Model file for the job. Use its own axes, mm. A direction names the side the tool comes from. Coordinates: 2 decimals unless noted, no trailing zeros. Order: outer loops, then holes, each group sorted by start corner. A loop starts at its lowest first (then second) coordinate and runs counter-clockwise, first axis right, second up.
from build123d import *

# Parameters (mm, degrees)
SKETCH_1_R              = 3
EXTRUDE_1_DEPTH         = 1.5
SHEET_START             = -1.5
SHEET_METAL_1_OUTLINE_R = 3
SHEET_METAL_1_DEPTH     = 1.5


# Read off the part's stored shape, not the designer's step: Преобразовать-Твердое тело1
with BuildPart() as part:
    # Sketch 1 → Бобышка-Вытянуть1 (new body)
    with BuildSketch(Plane.XY):
        with BuildLine():
            Line((-75, -160), (-75, 187.455080757))
            Line((-75, 187.455080757), (-302.165063509, 187.455080757))
            Line((-302.165063509, 187.455080757), (-346.732050808, 110.262794416))
            Line((-346.732050808, 110.262794416), (-364.052558883, 120.262794416))
            Line((-364.052558883, 120.262794416), (-374.052558883, 102.942286341))
            Line((-374.052558883, 102.942286341), (-356.732050808, 92.942286341))
            Line((-356.732050808, 92.942286341), (-401.299038106, 15.75))
            ThreePointArc((-401.299038106, 15.75), (-401.700961894, 14.25), (-401.299038106, 12.75))
            Line((-401.299038106, 12.75), (-376.299038106, -30.551270189))
            Line((-376.299038106, -30.551270189), (-392.320508076, -39.801270189))
            Line((-392.320508076, -39.801270189), (-382.320508076, -57.121778265))
            Line((-382.320508076, -57.121778265), (-366.299038106, -47.871778265))
            Line((-366.299038106, -47.871778265), (-241.299038106, -264.378129211))
            Line((-241.299038106, -264.378129211), (-257.320508076, -273.628129211))
            Line((-257.320508076, -273.628129211), (-247.320508076, -290.948637287))
            Line((-247.320508076, -290.948637287), (-231.299038106, -281.698637287))
            Line((-231.299038106, -281.698637287), (-203.75277675, -329.410161514))
            ThreePointArc((-203.75277675, -329.410161514), (-200.092522712, -333.070415552), (-195.092522712, -334.410161514))
            Line((-195.092522712, -334.410161514), (-149.133974596, -334.410161514))
            Line((-149.133974596, -334.410161514), (-149.133974596, -352.910161514))
            Line((-149.133974596, -352.910161514), (-129.133974596, -352.910161514))
            Line((-129.133974596, -352.910161514), (-129.133974596, -334.410161514))
            Line((-129.133974596, -334.410161514), (129.133974596, -334.410161514))
            Line((129.133974596, -334.410161514), (129.133974596, -352.910161514))
            Line((129.133974596, -352.910161514), (149.133974596, -352.910161514))
            Line((149.133974596, -352.910161514), (149.133974596, -334.410161514))
            Line((149.133974596, -334.410161514), (195.092522712, -334.410161514))
            ThreePointArc((195.092522712, -334.410161514), (200.092522712, -333.070415552), (203.75277675, -329.410161514))
            Line((203.75277675, -329.410161514), (231.299038106, -281.698637287))
            Line((231.299038106, -281.698637287), (247.320508076, -290.948637287))
            Line((247.320508076, -290.948637287), (257.320508076, -273.628129211))
            Line((257.320508076, -273.628129211), (241.299038106, -264.378129211))
            Line((241.299038106, -264.378129211), (366.299038106, -47.871778265))
            Line((366.299038106, -47.871778265), (382.320508076, -57.121778265))
            Line((382.320508076, -57.121778265), (392.320508076, -39.801270189))
            Line((392.320508076, -39.801270189), (376.299038106, -30.551270189))
            Line((376.299038106, -30.551270189), (401.299038106, 12.75))
            ThreePointArc((401.299038106, 12.75), (401.700961894, 14.25), (401.299038106, 15.75))
            Line((401.299038106, 15.75), (302.165063509, 187.455080757))
            Line((302.165063509, 187.455080757), (75, 187.455080757))
            Line((75, 187.455080757), (75, -160))
            ThreePointArc((75, -160), (0, -235), (-75, -160))
        make_face()
        with Locations((244.309773091, -277.663383249)):
            Circle(SKETCH_1_R, mode=Mode.SUBTRACT)
        with Locations((139.133974596, -343.660161514)):
            Circle(SKETCH_1_R, mode=Mode.SUBTRACT)
        with Locations((-139.133974596, -343.660161514)):
            Circle(SKETCH_1_R, mode=Mode.SUBTRACT)
        with Locations((-244.309773091, -277.663383249)):
            Circle(SKETCH_1_R, mode=Mode.SUBTRACT)
        with Locations((300, 10)):
            Circle(SKETCH_1_R, mode=Mode.SUBTRACT)
        with Locations((-300, 10)):
            Circle(SKETCH_1_R, mode=Mode.SUBTRACT)
        with Locations((-379.309773091, -43.836524227)):
            Circle(SKETCH_1_R, mode=Mode.SUBTRACT)
        with Locations((379.309773091, -43.836524227)):
            Circle(SKETCH_1_R, mode=Mode.SUBTRACT)
        with Locations((-360.392304845, 106.602540378)):
            Circle(SKETCH_1_R, mode=Mode.SUBTRACT)
    extrude(amount=EXTRUDE_1_DEPTH)

    # Sheet Metal 1 outline → Sheet Metal 1 (add)
    with BuildSketch(Plane.XY.offset(SHEET_START)):
        with BuildLine():
            Line((-149.133974596, -334.410161514), (-149.133974596, -352.910161514))
            Line((-149.133974596, -352.910161514), (-129.133974596, -352.910161514))
            Line((-129.133974596, -352.910161514), (-129.133974596, -334.410161514))
            Line((-129.133974596, -334.410161514), (129.133974596, -334.410161514))
            Line((129.133974596, -334.410161514), (129.133974596, -352.910161514))
            Line((129.133974596, -352.910161514), (149.133974596, -352.910161514))
            Line((149.133974596, -352.910161514), (149.133974596, -334.410161514))
            Line((149.133974596, -334.410161514), (195.092522712, -334.410161514))
            ThreePointArc((195.092522712, -334.410161514), (200.092522712, -333.070415552), (203.75277675, -329.410161514))
            Line((203.75277675, -329.410161514), (231.299038106, -281.698637287))
            Line((231.299038106, -281.698637287), (247.320508076, -290.948637287))
            Line((247.320508076, -290.948637287), (257.320508076, -273.628129211))
            Line((257.320508076, -273.628129211), (241.299038106, -264.378129211))
            Line((241.299038106, -264.378129211), (366.299038106, -47.871778265))
            Line((366.299038106, -47.871778265), (382.320508076, -57.121778265))
            Line((382.320508076, -57.121778265), (392.320508076, -39.801270189))
            Line((392.320508076, -39.801270189), (376.299038106, -30.551270189))
            Line((376.299038106, -30.551270189), (401.299038106, 12.75))
            ThreePointArc((401.299038106, 12.75), (401.700961894, 14.25), (401.299038106, 15.75))
            Line((401.299038106, 15.75), (302.165063509, 187.455080757))
            Line((302.165063509, 187.455080757), (75, 187.455080757))
            Line((75, 187.455080757), (75, -160))
            ThreePointArc((75, -160), (0, -235), (-75, -160))
            Line((-75, -160), (-75, 187.455080757))
            Line((-75, 187.455080757), (-302.165063509, 187.455080757))
            Line((-302.165063509, 187.455080757), (-346.732050808, 110.262794416))
            Line((-346.732050808, 110.262794416), (-364.052558883, 120.262794416))
            Line((-364.052558883, 120.262794416), (-374.052558883, 102.942286341))
            Line((-374.052558883, 102.942286341), (-356.732050808, 92.942286341))
            Line((-356.732050808, 92.942286341), (-401.299038106, 15.75))
            ThreePointArc((-401.299038106, 15.75), (-401.700961894, 14.25), (-401.299038106, 12.75))
            Line((-401.299038106, 12.75), (-376.299038106, -30.551270189))
            Line((-376.299038106, -30.551270189), (-392.320508076, -39.801270189))
            Line((-392.320508076, -39.801270189), (-382.320508076, -57.121778265))
            Line((-382.320508076, -57.121778265), (-366.299038106, -47.871778265))
            Line((-366.299038106, -47.871778265), (-241.299038106, -264.378129211))
            Line((-241.299038106, -264.378129211), (-257.320508076, -273.628129211))
            Line((-257.320508076, -273.628129211), (-247.320508076, -290.948637287))
            Line((-247.320508076, -290.948637287), (-231.299038106, -281.698637287))
            Line((-231.299038106, -281.698637287), (-203.75277675, -329.410161514))
            ThreePointArc((-203.75277675, -329.410161514), (-200.092522712, -333.070415552), (-195.092522712, -334.410161514))
            Line((-195.092522712, -334.410161514), (-149.133974596, -334.410161514))
        make_face()
        with Locations((-244.309773091, -277.663383249)):
            Circle(SHEET_METAL_1_OUTLINE_R, mode=Mode.SUBTRACT)
        with Locations((-139.133974596, -343.660161514)):
            Circle(SHEET_METAL_1_OUTLINE_R, mode=Mode.SUBTRACT)
        with Locations((139.133974596, -343.660161514)):
            Circle(SHEET_METAL_1_OUTLINE_R, mode=Mode.SUBTRACT)
        with Locations((244.309773091, -277.663383249)):
            Circle(SHEET_METAL_1_OUTLINE_R, mode=Mode.SUBTRACT)
        with Locations((-379.309773091, -43.836524227)):
            Circle(SHEET_METAL_1_OUTLINE_R, mode=Mode.SUBTRACT)
        with Locations((-300, 10)):
            Circle(SHEET_METAL_1_OUTLINE_R, mode=Mode.SUBTRACT)
        with Locations((-360.392304845, 106.602540378)):
            Circle(SHEET_METAL_1_OUTLINE_R, mode=Mode.SUBTRACT)
        with Locations((379.309773091, -43.836524227)):
            Circle(SHEET_METAL_1_OUTLINE_R, mode=Mode.SUBTRACT)
        with Locations((300, 10)):
            Circle(SHEET_METAL_1_OUTLINE_R, mode=Mode.SUBTRACT)
    extrude(amount=SHEET_METAL_1_DEPTH)


solid = part.part
Q1. Cut at D-D, the plane z = 0.75. Count the separate pieces of the cut face and the enclosed holes in it, plus the area to 3 significant figures.
Established:
separate pieces: 1
enclosed holes: 9
area: 274,000 mm2
Q2. Which spindle directions (+Z, -Z, +X, -X, +Y, -Y) get a long thin tool onto all of the face, cutting with end or side? Do faces 4 (the face through (-378.7, 54.89, -0.02)), 5 (the face through (1.65, -234.98, -0.02)), 6 (the face through (-217.72, -305.22, -0.02)). Say none if no direction does.
Established:
face 4: +Z, -Z, -X
face 5: +Z, -Z, +Y
face 6: +Z, -Z, -Y
Q3. Drop flat-ended pins along their axis: P1, Ø0.9, axis at y = -31.5, z = 0, coming from the +X side; P2, Ø0.9, axis at y = -343.5, z = 0.5, coming from the +X side; P3, Ø1.5, axis at x = 169, z = -0.5, coming from the -Y side. Give the stop position or say it passes through.
Established:
P1: stops at x = 378.72
P2: stops at x = 149.13
P3: stops at y = -334.41
Q4. Probe line 1 (Y direction, x = -110, z = -0.4); line 2 (X direction, y = -200, z = -0.6); line 3 (Y direction, x = -300, z = -0.55). List the from-to ranges inside material, lowest first.
Established:
line 1: y = -334.41 to 187.46
line 2: x = -278.47 to -63.44, 63.44 to 278.47
line 3: y = -162.71 to 7, 13 to 187.46
Q5. Cut at B-B, the plane x = -160.5. List the corners of the cut face in (y, z).
Established:
outline: (-334.41, -1.5) - (187.46, -1.5) - (187.46, 1.5) - (-334.41, 1.5) - close
Q6. Mould opens along Y. For faces 1 (the face through (217.33, -305.89, -0.02)), 2 (the face through (-95, -79, 1.5)), 3 (the face through (388.624, -9.204, -0.021)) say: pulls with the +Y half, pulls with the -Y half, needs draft (parallel to the pull), parting line crosses it, or undercut.
Established:
face 1: pulls with the -Y half
face 2: needs draft
face 3: undercut
Q7. Cut at C-C, the plane y = 147.5. List the corners of the cut face in (x, z), plus the area to 3 significant figures.
Established:
outline: (-325.23, -1.5) - (-75, -1.5) - (-75, 1.5) - (-325.23, 1.5) - close; (75, -1.5) - (325.23, -1.5) - (325.23, 1.5) - (75, 1.5) - close
area: 1,500 mm2
Q8. Cut at A-A, the plane y = 48.5. List the corners of the cut face in (x, z), plus the area to 3 significant figures.
Established:
outline: (-382.39, -1.5) - (-75, -1.5) - (-75, 1.5) - (-382.39, 1.5) - close; (75, -1.5) - (382.39, -1.5) - (382.39, 1.5) - (75, 1.5) - close
area: 1,840 mm2
